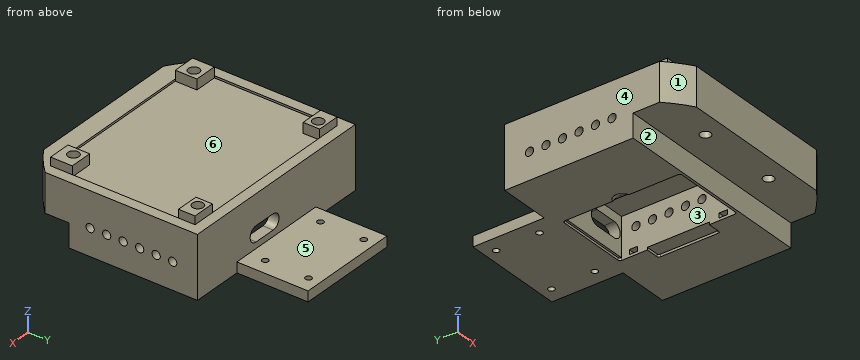
from build123d import *

# Parameters (mm, degrees)
RESSALTO_EXTRUS_O1_DEPTH   = 30
ESBO_O10_W                 = 112.198297798
ESBO_O10_H                 = 48.296192569
CORTE_EXTRUS_O6_DEPTH      = 25
CORTE_EXTRUS_O7_DEPTH      = 90.92898472
CORTE_EXTRUS_O7_DEPTH_BACK = 90.92898472
ESBO_O12_W                 = 36.72404194
ESBO_O12_H                 = 46.699624219
ESBO_O12_W_2               = 36.523308256
ESBO_O12_W_3               = 76.065965206
ESBO_O12_H_2               = 16.622456002
ESBO_O13_W                 = 35
ESBO_O13_H                 = 55
CORTE_EXTRUS_O8_DEPTH      = 20
CORTE_EXTRUS_O9_DEPTH      = 20
ESBO_O15_W                 = 90
ESBO_O15_H                 = 70
CORTE_EXTRUS_O10_DEPTH     = 1
ESBO_O16_W                 = 22.5
ESBO_O16_H                 = 55
CORTE_EXTRUS_O11_DEPTH     = 25
ESBO_O18_W                 = 90
ESBO_O18_H                 = 55
RESSALTO_EXTRUS_O2_DEPTH   = 3
ESBO_O19_W                 = 35
ESBO_O19_H                 = 55
CORTE_EXTRUS_O12_DEPTH     = 3
ESBO_O20_R                 = 2
CORTE_EXTRUS_O13_DEPTH     = 1500
ESBO_O21_W                 = 105.588179738
ESBO_O21_H                 = 28.353928622
CORTE_EXTRUS_O14_DEPTH     = 11.4
CORTE_EXTRUS_O15_DEPTH     = 10
ESBO_O23_R                 = 1.5
CORTE_EXTRUS_O16_DEPTH     = 6
ESBO_O29_W                 = 7
ESBO_O29_H                 = 30
CORTE_EXTRUS_O18_DEPTH     = 1.2
ESBO_O31_W                 = 2.3
ESBO_O31_H                 = 4
CORTE_EXTRUS_O19_DEPTH     = 4
ESBO_O33_W                 = 1
ESBO_O33_H                 = 6
CORTE_EXTRUS_O20_DEPTH     = 4
ESBO_O34_R                 = 2.5
CORTE_EXTRUS_O21_DEPTH     = 6
ESBO_O35_W                 = 11
ESBO_O35_H                 = 8
ESBO_O35_H_2               = 10.5
RESSALTO_EXTRUS_O3_DEPTH   = 5
ESBO_O36_R                 = 2.65
CORTE_EXTRUS_O22_DEPTH     = 4.7
ESBO_O38_W                 = 36
ESBO_O38_H                 = 57
CORTE_EXTRUS_O23_DEPTH     = 1.2
FILETE4_R                  = 1
FILETE5_R                  = 1
FILETE6_R                  = 1
ESBO_O40_R                 = 4.036676011
CORTE_EXTRUS_O25_DEPTH     = 1
FILETE9_R                  = 4


with BuildPart() as part:
    # Esboço1 → Ressalto-extrusão1 (new body)
    with BuildSketch(Plane.XY):
        with BuildLine():
            Line((-49.381601242, -49.613077498), (-49.381601242, 49.613077498))
            ThreePointArc((-49.381601242, 49.613077498), (0.883684189, 69.994421937), (50.618398758, 48.350570908))
            Line((50.618398758, 48.350570908), (50.618398758, -48.350570908))
            ThreePointArc((50.618398758, -48.350570908), (0.883684189, -69.994421937), (-49.381601242, -49.613077498))
        make_face()
    extrude(amount=RESSALTO_EXTRUS_O1_DEPTH)

    # Esboço10 → Corte-extrusão6 (cut)
    with BuildSketch(Plane.XY.offset(30)):
        with Locations((0, 49.593404353)):
            Rectangle(ESBO_O10_W, ESBO_O10_H)
    extrude(amount=-CORTE_EXTRUS_O6_DEPTH, mode=Mode.SUBTRACT)

    # Esboço12 → Corte-extrusão7 (cut, two sides: drawn at the far end of the back side and taken through both)
    with BuildSketch(Plane.XY.offset(5).offset(-CORTE_EXTRUS_O7_DEPTH_BACK)):
        with Locations((-42.743622212, 48.795120178)):
            Rectangle(ESBO_O12_W, ESBO_O12_H)
        with Locations((43.880052886, 48.795120178)):
            Rectangle(ESBO_O12_W_2, ESBO_O12_H)
        with Locations((0, -67.077648977)):
            Rectangle(ESBO_O12_W_3, ESBO_O12_H_2)
    extrude(amount=CORTE_EXTRUS_O7_DEPTH + CORTE_EXTRUS_O7_DEPTH_BACK, mode=Mode.SUBTRACT)

    # Esboço13 → Corte-extrusão8 (cut)
    with BuildSketch(Plane(origin=(0, 0, 0), x_dir=(-1, 0, 0), z_dir=(0, 0, -1))):
        with Locations((-0.618398758, -7.054691932)):
            Rectangle(ESBO_O13_W, ESBO_O13_H)
    extrude(amount=-CORTE_EXTRUS_O8_DEPTH, mode=Mode.SUBTRACT)

    # Esboço14 → Corte-extrusão9 (cut)
    with BuildSketch(Plane(origin=(0, 25.445308068, 0), x_dir=(1, 0, 0), z_dir=(0, 1, 0))):
        with BuildLine():
            Line((2.653109582, -7.998476533), (13.483040952, -7.998476533))
            ThreePointArc((13.483040952, -7.998476533), (17.204697231, -11.720132813), (13.483040952, -15.441789092))
            Line((13.483040952, -15.441789092), (2.653109582, -15.441789092))
            ThreePointArc((2.653109582, -15.441789092), (-1.068546697, -11.720132813), (2.653109582, -7.998476533))
        make_face()
    extrude(amount=-CORTE_EXTRUS_O9_DEPTH, mode=Mode.SUBTRACT)

    # Esboço15 → Corte-extrusão10 (cut)
    with BuildSketch(Plane.XY.offset(30)):
        with Locations((0.618398758, -14.554691932)):
            Rectangle(ESBO_O15_W, ESBO_O15_H)
    extrude(amount=-CORTE_EXTRUS_O10_DEPTH, mode=Mode.SUBTRACT)

    # Esboço16 → Corte-extrusão11 (cut)
    with BuildSketch(Plane(origin=(0, 0, 0), x_dir=(-1, 0, 0), z_dir=(0, 0, -1))):
        with Locations((-34.368398758, -7.054691932)):
            Rectangle(ESBO_O16_W, ESBO_O16_H)
        with Locations((33.131601242, -7.054691932)):
            Rectangle(ESBO_O16_W, ESBO_O16_H)
    extrude(amount=-CORTE_EXTRUS_O11_DEPTH, mode=Mode.SUBTRACT)

    # Esboço18 → Ressalto-extrusão2 (add)
    with BuildSketch(Plane(origin=(0, 0, 0), x_dir=(-1, 0, 0), z_dir=(0, 0, -1))):
        with Locations((-0.618398758, -7.054691932)):
            Rectangle(ESBO_O18_W, ESBO_O18_H)
    extrude(amount=-RESSALTO_EXTRUS_O2_DEPTH)

    # Esboço19 → Corte-extrusão12 (cut)
    with BuildSketch(Plane(origin=(0, 0, 0), x_dir=(-1, 0, 0), z_dir=(0, 0, -1))):
        with Locations((-0.618398758, -7.054691932)):
            Rectangle(ESBO_O19_W, ESBO_O19_H)
    extrude(amount=-CORTE_EXTRUS_O12_DEPTH, mode=Mode.SUBTRACT)

    # Esboço20 → Corte-extrusão13 (cut)
    with BuildSketch(Plane(origin=(50.618398758, 0, 0), x_dir=(0, 0, -1), z_dir=(1, 0, 0))):
        with Locations((-13, 5.445308068)):
            Circle(ESBO_O20_R)
        with Locations((-13, -2.554691932)):
            Circle(ESBO_O20_R)
        with Locations((-13, 13.445308068)):
            Circle(ESBO_O20_R)
        with Locations((-13, -10.554691932)):
            Circle(ESBO_O20_R)
        with Locations((-13, -18.554691932)):
            Circle(ESBO_O20_R)
        with Locations((-13, -26.554691932)):
            Circle(ESBO_O20_R)
    extrude(amount=-CORTE_EXTRUS_O13_DEPTH, mode=Mode.SUBTRACT)

    # Esboço21 → Corte-extrusão14 (cut)
    with BuildSketch(Plane(origin=(0, 0, 0), x_dir=(-1, 0, 0), z_dir=(0, 0, -1))):
        with Locations((2.175691111, -50.943385287)):
            Rectangle(ESBO_O21_W, ESBO_O21_H)
    extrude(amount=-CORTE_EXTRUS_O14_DEPTH, mode=Mode.SUBTRACT)

    # Esboço22 → Corte-extrusão15 (cut)
    with BuildSketch(Plane.XY.offset(5)):
        Polygon((-29.980530995, 70.945308068), (31.249974599, 70.942177058), (31.249974599, 59.945308068), (-29.980530995, 59.945308068), align=None)
    extrude(amount=-CORTE_EXTRUS_O15_DEPTH, mode=Mode.SUBTRACT)

    # Esboço23 → Corte-extrusão16 (cut)
    with BuildSketch(Plane.XY.offset(5)):
        with Locations((-16.881601242, 54.445308068)):
            Circle(ESBO_O23_R)
        with Locations((-16.881601242, 33.445308068)):
            Circle(ESBO_O23_R)
        with Locations((18.118398758, 33.445308068)):
            Circle(ESBO_O23_R)
        with Locations((18.118398758, 54.445308068)):
            Circle(ESBO_O23_R)
    extrude(amount=-CORTE_EXTRUS_O16_DEPTH, mode=Mode.SUBTRACT)

    # Esboço29 → Corte-extrusão18 (cut)
    with BuildSketch(Plane(origin=(0, 0, 0), x_dir=(-1, 0, 0), z_dir=(0, 0, -1))):
        with Locations((-21.618398758, -7.054691932)):
            Rectangle(ESBO_O29_W, ESBO_O29_H)
    extrude(amount=-CORTE_EXTRUS_O18_DEPTH, mode=Mode.SUBTRACT)

    # Esboço31 → Corte-extrusão19 (cut)
    with BuildSketch(Plane.ZY.offset(-18.118398758)):
        with Locations((2.35, 14.688444073)):
            Rectangle(ESBO_O31_W, ESBO_O31_H)
        with Locations((2.35, -28.797827937)):
            Rectangle(ESBO_O31_W, ESBO_O31_H)
    extrude(amount=-CORTE_EXTRUS_O19_DEPTH, mode=Mode.SUBTRACT)

    # Esboço33 → Corte-extrusão20 (cut)
    with BuildSketch(Plane(origin=(-16.881601242, 0, 0), x_dir=(0, 0, -1), z_dir=(1, 0, 0))):
        with Locations((-2, -6.723435912)):
            Rectangle(ESBO_O33_W, ESBO_O33_H)
    extrude(amount=-CORTE_EXTRUS_O20_DEPTH, mode=Mode.SUBTRACT)

    # Esboço34 → Corte-extrusão21 (cut)
    with BuildSketch(Plane(origin=(0, 0, 11.4), x_dir=(-1, 0, 0), z_dir=(0, 0, -1))):
        with Locations((20, -49.366420976)):
            Circle(ESBO_O34_R)
        with Locations((-20, -49.366420976)):
            Circle(ESBO_O34_R)
    extrude(amount=-CORTE_EXTRUS_O21_DEPTH, mode=Mode.SUBTRACT)

    # Esboço35 → Ressalto-extrusão3 (add)
    with BuildSketch(Plane.XY.offset(29)):
        with Locations((-38.881601242, 16.445308068)):
            Rectangle(ESBO_O35_W, ESBO_O35_H)
        with Locations((40.118398758, 16.445308068)):
            Rectangle(ESBO_O35_W, ESBO_O35_H)
        with Locations((40.118398758, -44.304691932)):
            Rectangle(ESBO_O35_W, ESBO_O35_H_2)
        with Locations((-38.881601242, -44.304691932)):
            Rectangle(ESBO_O35_W, ESBO_O35_H_2)
    extrude(amount=RESSALTO_EXTRUS_O3_DEPTH)

    # Esboço36 → Corte-extrusão22 (cut)
    with BuildSketch(Plane.XY.offset(34)):
        with Locations((-37.531601242, 16.595308068)):
            Circle(ESBO_O36_R)
        with Locations((38.768398758, 16.595308068)):
            Circle(ESBO_O36_R)
        with Locations((38.768398758, -43.704691932)):
            Circle(ESBO_O36_R)
        with Locations((-37.531601242, -43.704691932)):
            Circle(ESBO_O36_R)
    extrude(amount=-CORTE_EXTRUS_O22_DEPTH, mode=Mode.SUBTRACT)

    # Esboço38 → Corte-extrusão23 (cut)
    with BuildSketch(Plane(origin=(0, 0, 0), x_dir=(-1, 0, 0), z_dir=(0, 0, -1))):
        with Locations((-0.118398758, -7.054691932)):
            Rectangle(ESBO_O38_W, ESBO_O38_H)
    extrude(amount=-CORTE_EXTRUS_O23_DEPTH, mode=Mode.SUBTRACT)

    # Filete4
    filete4_edges = [part.edges().sort_by_distance(p)[0] for p in [
        (-17.881601242, 21.445308068, 0.6),
    ]]
    fillet(filete4_edges, radius=FILETE4_R)

    # Filete5
    filete5_edges = [part.edges().sort_by_distance(p)[0] for p in [
        (18.118398758, -35.554691932, 0.6),
        (-17.881601242, -35.554691932, 0.6),
        (18.118398758, 21.445308068, 0.6),
    ]]
    fillet(filete5_edges, radius=FILETE5_R)

    # Filete6
    filete6_edges = [part.edges().sort_by_distance(p)[0] for p in [
        (25.118398758, -22.054691932, 0.6),
        (25.118398758, 7.945308068, 0.6),
    ]]
    fillet(filete6_edges, radius=FILETE6_R)

    # Esboço40 → Corte-extrusão25 (cut)
    with BuildSketch(Plane(origin=(0, 0, 0), x_dir=(-1, 0, 0), z_dir=(0, 0, -1))):
        with Locations((16.881601242, -6.723435912)):
            Circle(ESBO_O40_R)
    extrude(amount=-CORTE_EXTRUS_O25_DEPTH, mode=Mode.SUBTRACT)

    # Filete9
    # the kernel refuses this fillet: 4 mm, written as the material it adds along each edge
    with BuildSketch(Plane(origin=(-16.881601242, -6.723435912, 1), x_dir=(0.9837182515450056, 0.17971756057001487, 0), z_dir=(0.17971756057001487, -0.9837182515450056, 0))) as filete9_piece_1_section:
        with BuildLine():
            CenterArc((1.3909247, -4), FILETE9_R, 48.590377891, 41.409622109)
            Line((1.3909247, 0), (1.3909247, 0.08))
            Line((1.3909247, 0.08), (4.036676011, 0.08))
            Line((4.036676011, 0.08), (4.116676011, 0))
            ThreePointArc((4.116676011, 0), (4.116676011, -0.5), (4.089591037, -0.94))
            Line((4.089591037, -0.94), (4.036676011, -1))
        make_face()
    filete9_piece_1 = revolve(axis=Axis((-16.881601242, -6.723435912, 1), (0, 0, 1)), revolution_arc=339.293382111, mode=Mode.PRIVATE)
    filete9_piece_1 = split(filete9_piece_1, bisect_by=Plane(origin=(-17.881601242, -6.723435912, 1), z_dir=(-1, 0, 0)), keep=Keep.TOP, mode=Mode.PRIVATE)
    add(filete9_piece_1)


solid = part.part
Read the model definition and answer for the solid it produces. Units are mm, in the model's axes. Face numbers are marked on the shaded views. A direction names the side the tool comes from. Coordinates: 2 decimals unless noted, no trailing zeros. Order: outer loops, then holes, each group sorted by start corner. A loop starts at its lowest first (then second) coordinate and runs counter-clockwise, first axis right, second up. Notation, with made-up numbers: (4, 59) - (56, 59) arc R16 ccw to (56, 75) - close; hole circle Ø9 at (22, -25.5). An arc over 180 degrees is marked (long way). Use one line per item in the form item = value.
(1) Straight lines are drawn through the part: L1, parallel to X at y = 4, z = 4; L2, parallel to Z at x = 32, y = 5; L3, parallel to Y at x = -7.5, z = 2. For each, find the intervals that lie inside material, in ascending order.
Computed values:
L1 = -49.38 to -44.38, -21.88 to -16.88, 18.12 to 23.12, 45.62 to 50.62
L2 = 0 to 3, 25 to 29
L3 = -36.77 to -34.55, 20.45 to 59.95
(2) Section C-C, the plane z = 13 is taken. Give the number of separate pieces and of enclosed holes in the cut face, then the cut area to 3 significant figures.
Computed values:
separate_pieces = 23
enclosed_holes = 2
area = 3,300 mm²
(3) Section A-A, the plane x = 6.5 is taken. Give the vertices of the cut face in (y, z).
Computed values:
outline = (-58.77, 11.4) - (-36.77, 11.4) - (-36.77, 0) - (-35.55, 0) - (-35.55, 1.2) - (-34.55, 1.2) - (-34.55, 20) - (20.45, 20) - (20.45, 15.44) - (25.45, 15.44) - (25.45, 30) - (20.45, 30) - (20.45, 29) - (-49.55, 29) - (-49.55, 30) - (-58.77, 30) - close; (20.45, 1.2) - (21.45, 1.2) - (21.45, 0) - (59.95, 0) - (59.95, 5) - (25.45, 5) - (25.45, 8) - (20.45, 8) - close
(4) Which of the six approach directions +Z, -Z, +X, -X, +Y, -Y give full straight-line access (tool end or side, diameter ignored) to the marked faces 1, 2 and 3?
Computed values:
face_1 = +Z, -Z, -X, -Y
face_2 = -Z, +X, -X, -Y
face_3 = -Z
(5) Section B-B, the plane x = -10.5 is taken. Give the vertices of the cut face in (y, z), then the cut area to 3 significant figures.
Computed values:
outline = (-58.77, 11.4) - (-36.77, 11.4) - (-36.77, 0) - (-35.55, 0) - (-35.55, 1.2) - (-34.55, 1.2) - (-34.55, 20) - (20.45, 20) - (20.45, 1.2) - (21.45, 1.2) - (21.45, 0) - (59.95, 0) - (59.95, 5) - (25.45, 5) - (25.45, 30) - (20.45, 30) - (20.45, 29) - (-49.55, 29) - (-49.55, 30) - (-58.77, 30) - close
area = 1,280 mm²
(6) Given pin 1 Ø1.5 at (x, z) = (-16.5, 11.5) entering from +Y; pin 2 Ø12 at (x, y) = (7, 14) entering from -Z; pin 3 Ø1.2 at (y, z) = (16, 32.5) entering from -X, each flat-ended and moving along its own axis, determine where each tip first touches the part or whether it passes through.
Computed values:
pin_1 = 25.45
pin_2 = 20
pin_3 = -44.38
(7) For a pull along X with two mould halves and no side action, classify the marked faces 4, 5 and 6 as pulls with the +X half, pulls with the -X half, needs draft (parallel to the pull), parting line crosses it, or undercut.
Computed values:
face_4 = pulls with the -X half
face_5 = needs draft
face_6 = undercut
